Verification items for the finished model (mm, model axes). A direction names the side the tool comes from. Give positions to 0.01 mm unless a question says otherwise; leave off trailing zeros. Write each loop counter-clockwise with the first axis right and the second up, starting at its lowest first coordinate (ties: lowest second). Pieces come first, ordered by that corner, then holes. Notation, with made-up numbers: M -14.75,-9.5 L 22.25,-9.5 A31 cw 22.25,20.5 Z; hole C -21.5,83 d7. An arc over 180 degrees is marked long. Answer as a JSON object with one key per item and string values.
```python
from build123d import *

# Parameters (mm, degrees)
F1_R     = 7.5
F1_W     = 30
F1_H     = 10
F2_DEPTH = 20


with BuildPart() as f2:
    # F1 (on face) → F2 (new body, symmetric)
    with BuildSketch(Plane.XZ):
        Polygon((-60, 30), (-60, -20), (0, -20), (15, -20), (15, 0), (15, 30), align=None)
        Circle(F1_R, mode=Mode.SUBTRACT)
        with Locations((-35, 15)):
            Rectangle(F1_W, F1_H, mode=Mode.SUBTRACT)
    extrude(amount=F2_DEPTH, both=True)


solid = f2.part
```
1) Access from +Z, -Z, +X, -X, +Y, -Y to the whole of each face (thin tool, end or side, straight path). Record for faces 1 (the face through (-50, 0, 15)), 2 (the face through (-23, -20, 5)).
Completed:
{"face 1": "+Y, -Y", "face 2": "+Z, -Z, +X, -X, -Y"}
2) Release check for a two-part mould opening along X. For faces 3 (the face through (-20, 0, 15)), 4 (the face through (15, 0, 5)), 5 (the face through (-35, 0, 10)), 6 (the face through (-22, 0, 30)) record: pulls with the +X half, pulls with the -X half, needs draft (parallel to the pull), parting line crosses it, or undercut.
Completed:
{"face 3": "undercut", "face 4": "pulls with the +X half", "face 5": "undercut", "face 6": "needs draft"}
3) Thickness scan on L1, parallel to Z at x = 0, y = 11; L2, parallel to Z at x = -40, y = 13; L3, parallel to X at y = 16, z = 19. Record the ranges inside material, lowest first.
Completed:
{"L1": "z = -20 to -7.5, 7.5 to 30", "L2": "z = -20 to 10, 20 to 30", "L3": "x = -60 to -50, -20 to 15"}
4) Section check A-A on z = 17. Record the boundary of the cut face in (x, y), and give its area (3 significant figures).
Completed:
{"outline": "M -60,-20 L -50,-20 L -50,20 L -60,20 Z; M -20,-20 L 15,-20 L 15,20 L -20,20 Z", "area": "1,800 mm2"}
5) Section check C-C on y = -12.5. Record the boundary of the cut face in (x, z).
Completed:
{"outline": "M -60,-20 L 15,-20 L 15,30 L -60,30 Z; hole M -50,10 L -20,10 L -20,20 L -50,20 Z; hole C 0,0 d15"}
6) Section check B-B on x = 0. Record the boundary of the cut face in (y, z).
Completed:
{"outline": "M -20,-20 L 20,-20 L 20,-7.5 L -20,-7.5 Z; M -20,7.5 L 20,7.5 L 20,30 L -20,30 Z"}
